```python
from build123d import *

# Parameters (mm, degrees)
BOSS_EXTRUDE1_DEPTH = 311.15
SKETCH2_W           = 38.1
SKETCH2_H           = 88.9
CUT_EXTRUDE1_DEPTH  = 354.914009094


with BuildPart() as part:
    # Sketch1 → Boss-Extrude1 (new, symmetric)
    with BuildSketch(Plane.XY):
        Polygon((0, 0), (0, -3.666174209), (-146.05, 80.655832606), (-146.05, 84.322006815), align=None)
    extrude(amount=BOSS_EXTRUDE1_DEPTH, both=True)

    # Sketch2 → Cut-Extrude1 (cut, through all)
    with BuildSketch(Plane(origin=(0, 0, 0), x_dir=(1, 0, 0), z_dir=(0, 1, 0))):
        with Locations((-127, -266.7)):
            Rectangle(SKETCH2_W, SKETCH2_H)
        with Locations((-127, 266.7)):
            Rectangle(SKETCH2_W, SKETCH2_H)
    extrude(amount=CUT_EXTRUDE1_DEPTH, mode=Mode.SUBTRACT)


solid = part.part
```
For this review, take the finished solid that the model builds, in its own axes (mm). Coordinates: 2 decimals unless noted, no trailing zeros. Order: outer loops, then holes, each group sorted by start corner. A loop starts at its lowest first (then second) coordinate and runs counter-clockwise, first axis right, second up. Notation, with made-up numbers: (1.25, -4) - (14.25, -4) arc R36 ccw to (14.25, 34) - close; hole circle Ø8 at (60.25, 80). An arc over 180 degrees is marked (long way). Answer as a JSON object with one key per item and string values. Group by question number.
1. We need section A-A on z = 250. State the section outline as (x, y) points.
2. We need section B-B on y = 25.5. State the section outline as (x, z) points.
3. For probe 1 along X at (y, z) = (26.5, 263); probe 2 along Y at (x, z) = (-13.5, 99); probe 3 along Y at (x, z) = (-138.5, 4), list the stretches that pass through material, from the lowest coordinate up.
4. Clearance check with flat-ended pins moving along their axes: P1, Ø6, axis at x = -53.5, z = -215, coming from the +Y side; P2, Ø5, axis at y = 5, z = 40, coming from the +X side; P3, Ø1.5, axis at y = 43, z = -142, coming from the -X side. State where each tip first meets the part, or that it passes through.
Final values:
{
 "1": {"outline": "(-107.95, 58.66) - (0, -3.67) - (0, 0) - (-107.95, 62.32) - close"},
 "2": {"outline": "(-50.52, -311.15) - (-44.17, -311.15) - (-44.17, 311.15) - (-50.52, 311.15) - close"},
 "3": {"probe 1": "-52.25 to -45.9", "probe 2": "4.13 to 7.79", "probe 3": "76.3 to 79.96"},
 "4": {"P1": "y = 32.62", "P2": "x = -4.33", "P3": "x = -82.13"}
}
